Design review of the part shown in the three views and the two pictorial views. Dimensions are in mm from the part's minimum x, y and z. Coordinates: 2 decimals unless noted, no trailing zeros. Loops run counter-clockwise (first coordinate to the right, second up) from the corner with the lowest first, then second, coordinate; pieces in that order, holes last. Notation, with made-up numbers: (11, 51.5) -> (28, 51.5) arc R15 cw to (28, 69.5) -> close; hole circle Ø7 at (58.25, 10.25). An arc over 180 degrees is marked (long way). One line per item, written item: value.
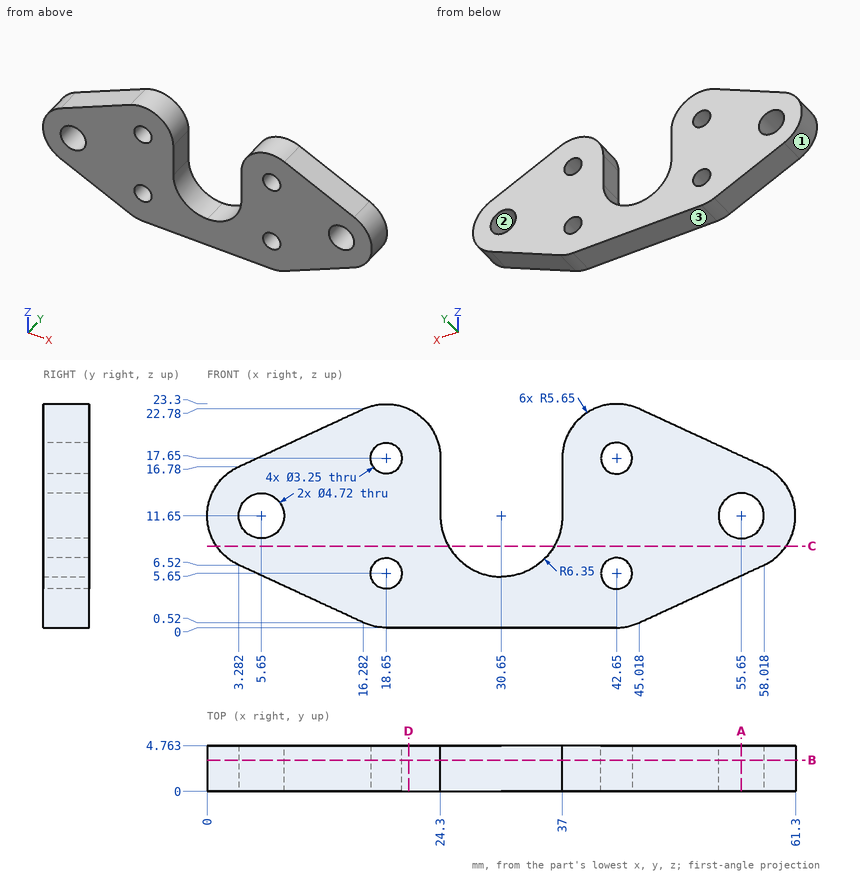
1. Take a section at C-C, the plane z = 8.5. Give the boundary of the cut face in (x, y), and give its area (3 significant figures).
Return value:
outline: (0.96, 0) -> (25.14, 0) -> (25.14, 4.76) -> (0.96, 4.76) -> close; (36.16, 0) -> (60.34, 0) -> (60.34, 4.76) -> (36.16, 4.76) -> close
area: 230 mm2
2. Take a section at D-D, the plane x = 21. Give the boundary of the cut face in (y, z).
Return value:
outline: (0, 0) -> (4.76, 0) -> (4.76, 22.79) -> (0, 22.79) -> close
3. The part is to be moulded in two halves that separate along X. For the marked faces 1, 2 and 3, say which applies: pulls with the +X half, pulls with the -X half, needs draft (parallel to the pull), parting line crosses it, or undercut.
Return value:
face 1: pulls with the -X half
face 2: undercut
face 3: needs draft
4. Take a section at A-A, the plane x = 55.65. Give the boundary of the cut face in (y, z), and give its area (3 significant figures).
Return value:
outline: (0, 5.43) -> (4.76, 5.43) -> (4.76, 9.29) -> (0, 9.29) -> close; (0, 14.01) -> (4.76, 14.01) -> (4.76, 17.87) -> (0, 17.87) -> close
area: 36.8 mm2
5. Take a section at B-B, the plane y = 3.25. Give the number of separate pieces and of enclosed holes in the cut face, and give its area (3 significant figures).
Return value:
separate pieces: 1
enclosed holes: 6
area: 846 mm2
6. To check wall thickness, follow probe 1 along Z at (x, y) = (18.65, 3.1) (1 decimal); probe 2 along X at (y, z) = (3.6, 4.5) (1 decimal); probe 3 along X at (y, z) = (3.5, 13) (1 decimal). State the ranges of each line that lie inside material, in increasing order. Write a range as from..to.
Return value:
probe 1: z = 0..4, 7.3..16, 19.3..23.3
probe 2: x = 7.7..17.5, 19.8..41.5, 43.8..53.6
probe 3: x = 0.2..3.7, 7.6..24.3, 37..53.7, 57.6..61.1
7. Insertion check: pin 1 Ø2 at (y, z) = (2, 19) entering from +X (1 decimal); pin 2 Ø1 at (x, y) = (15.5, 1.5) entering from -Z; pin 3 Ø2 at (y, z) = (4, 20) entering from +X (1 decimal). Each pin has a flat end and moves straight along its axis. Give the tip position at first contact, or say it passes through.
Return value:
pin 1: stops at x = 55.4
pin 2: stops at z = 0.65
pin 3: stops at x = 53.2
